Source: three-view drawing plus pictorial views. Frame: mm from the lowest corner of the part. Round coordinates to 2 decimals unless told otherwise and drop trailing zeros. Order: outer loops, then holes, each group sorted by start corner. A loop starts at its lowest first (then second) coordinate and runs counter-clockwise, first axis right, second up. Notation, with made-up numbers: (-22.5, 46) -> (28.5, 46) arc R37 cw to (28.5, 82) -> close; hole circle Ø7 at (-4.5, -30.5). An arc over 180 degrees is marked (long way). Use a Markdown table: item, result.
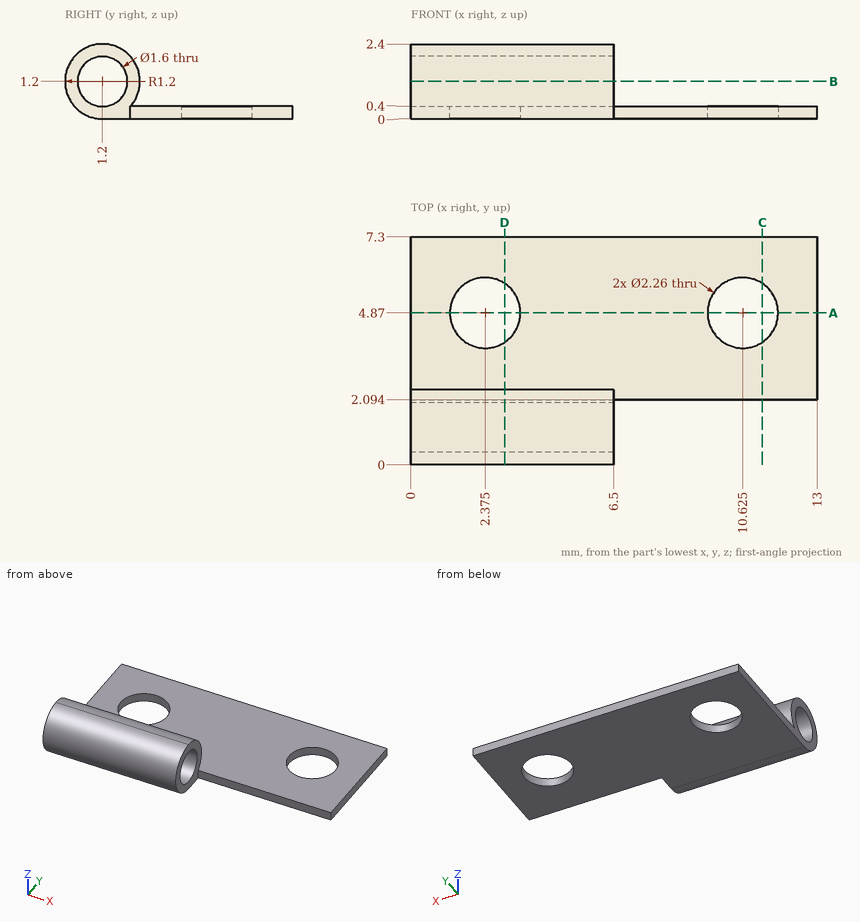
1) Cut plane B-B on z = 1.2. Return loops of the section in (x, y).
Results found:
| item | result |
|---|---|
| outline | (0, 0) -> (6.5, 0) -> (6.5, 0.4) -> (0, 0.4) -> close; (0, 2) -> (6.5, 2) -> (6.5, 2.4) -> (0, 2.4) -> close |
2) Cut plane D-D on x = 3. Return loops of the section in (y, z) (1 decimal).
Results found:
| item | result |
|---|---|
| outline | (1.2, 0) -> (3.9, 0) -> (3.9, 0.4) -> (2.1, 0.4) arc R1.2 ccw (long way) to start; (5.8, 0) -> (7.3, 0) -> (7.3, 0.4) -> (5.8, 0.4) -> close; hole circle Ø1.6 at (1.2, 1.2) |
3) Pin query (flat end, axial travel): pin 1 Ø1.5 at (x, y) = (1.5, 4.5) entering from -Z. Return the tip coordinate at first contact, or that it passes through.
Results found:
| item | result |
|---|---|
| pin 1 | stops at z = 0 |
4) Cut plane C-C on x = 11.25. Return loops of the section in (y, z) (1 decimal).
Results found:
| item | result |
|---|---|
| outline | (2.1, 0) -> (3.9, 0) -> (3.9, 0.4) -> (2.1, 0.4) -> close; (5.8, 0) -> (7.3, 0) -> (7.3, 0.4) -> (5.8, 0.4) -> close |
5) Cut plane A-A on y = 4.87. Return loops of the section in (x, z) (1 decimal).
Results found:
| item | result |
|---|---|
| outline | (0, 0) -> (1.2, 0) -> (1.2, 0.4) -> (0, 0.4) -> close; (3.5, 0) -> (9.5, 0) -> (9.5, 0.4) -> (3.5, 0.4) -> close; (11.8, 0) -> (13, 0) -> (13, 0.4) -> (11.8, 0.4) -> close |
6) Line query: L1, parallel to Z at x = 9.25, y = 5; L2, parallel to Y at x = 4, z = 1.45 (1 decimal); L3, parallel to Y at x = 2.25, z = 1.5. Output: solid intervals per line, ascending. Write a range as [from, to].
Results found:
| item | result |
|---|---|
| L1 | z = [0, 0.4] |
| L2 | y = [0, 0.4], [2, 2.4] |
| L3 | y = [0.04, 0.46], [1.94, 2.36] |
